Here's how the part is built. I have some questions about the finished solid (model axes, mm). A direction names the side the tool comes from. Give positions to 0.01 mm unless a question says otherwise; leave off trailing zeros. Order: outer loops, then holes, each group sorted by start corner. A loop starts at its lowest first (then second) coordinate and runs counter-clockwise, first axis right, second up.
from build123d import *
from build123d import SkipClean  # not in build123d's __all__

# Parameters (mm, degrees)
F2_R      = 1.25
F3_DEPTH  = 8.001
F5_R      = 1.25
F5_R_2    = 0.9
F6_DEPTH  = 3.2
F7_W      = 1
F7_H      = 4
F8_DEPTH  = 8
F9_R      = 0.9
F10_DEPTH = 2


with BuildPart() as f1:
    # F0 (on Right) → F1 (revolve)
    with BuildSketch(Plane.YZ):
        with BuildLine():
            Line((5, -0.8), (5, 0))
            ThreePointArc((5, 0), (3.5355339059, 3.5355339059), (0, 5))
            Line((0, 5), (0, -8))
            Line((0, -8), (1.7, -8))
            Line((1.7, -8), (1.7, 0))
            Line((1.7, 0), (4.6, 0))
            Line((4.6, 0), (4.6, -0.8))
            Line((4.6, -0.8), (5, -0.8))
        make_face()
    revolve(axis=Axis((0, 0, -1.5), (0, 0, -1)))

    # F2 (on Top) → F3 (cut, through all)
    with BuildSketch(Plane.XY):
        Circle(F2_R)
    extrude(amount=-F3_DEPTH, mode=Mode.SUBTRACT)

    # F5 (on face) → F6 (join)
    with BuildSketch(Plane(origin=(0, 0, 0), x_dir=(1, 0, 0), z_dir=(0, 0, -1))):
        Circle(F5_R)
        Circle(F5_R_2, mode=Mode.SUBTRACT)
    extrude(amount=F6_DEPTH)

    # F7 (on face) → F8 (cut, through all)
    with BuildSketch(Plane(origin=(0, 0, -8), x_dir=(1, 0, 0), z_dir=(0, 0, -1))):
        Rectangle(F7_W, F7_H)
    extrude(amount=-F8_DEPTH, mode=Mode.SUBTRACT)

    # F9 (on face) → F10 (cut)
    with BuildSketch(Plane(origin=(0, 0, 0), x_dir=(1, 0, 0), z_dir=(0, 0, -1))):
        Circle(F9_R)
    with SkipClean():  # cleaning this boolean's faces spoils the solid; the shape is the same uncleaned
        extrude(amount=-F10_DEPTH, mode=Mode.SUBTRACT)


solid = f1.part
Q1. I need wall thicknesses on L1, parallel to X at y = 0, z = -0.3; L2, parallel to X at y = 0, z = 0.65; L3, parallel to Y at x = 1.25, z = -0.25. Which ranges of each line are inside material? Lowest first, please.
Filled sheet:
L1: x = -5 to -4.6, -1.7 to -0.9, 0.9 to 1.7, 4.6 to 5
L2: x = -4.96 to -0.9, 0.9 to 4.96
L3: y = -4.84 to -4.43, -1.15 to 1.15, 4.43 to 4.84
Q2. If we section it at A-A on z = -1.5: List the corners of the cut face in (x, y) for me.
Filled sheet:
outline: (-0.5, -1.62) - (-0.5, -0.75) arc R0.9 cw to (-0.5, 0.75) - (-0.5, 1.62) arc R1.7 ccw to start; (0.5, -1.62) arc R1.7 ccw to (0.5, 1.62) - (0.5, 0.75) arc R0.9 cw to (0.5, -0.75) - close
Q3. If we section it at D-D on z = 1.25: List the corners of the cut face in (x, y) for me, plus the area to 3 significant figures.
Filled sheet:
outline: circle Ø9.68 at (0, 0); hole circle Ø1.8 at (0, 0)
area: 71.1 mm2
Q4. I'm going to push flat-ended pins straight in: P1, Ø0.8, axis at x = 1, y = -0.5, coming from the -Z side; P2, Ø0.7, axis at y = -1, z = -6, coming from the -X side; P3, Ø3, axis at x = -4, y = -3.5, coming from the +Z side; P4, Ø0.9, axis at x = -0.5, y = 0.5, coming from the -Z side. Where does each tip first touch, or does it pass through?
Filled sheet:
P1: stops at z = -8
P2: stops at x = -1.57
P3: stops at z = 3.23
P4: stops at z = -3.2
Q5. If we section it at B-B on x = 0: List the corners of the cut face in (y, z) for me.
Filled sheet:
outline: (-5, -0.8) - (-4.6, -0.8) - (-4.6, 0) - (-0.9, 0) - (-0.9, 2) - (0.9, 2) - (0.9, 0) - (4.6, 0) - (4.6, -0.8) - (5, -0.8) - (5, 0) arc R5 ccw to (-5, 0) - close
Q6. Thinking about a two-plate mould opening in Y: for faces 1 (the face through (1.25, -0.02, -5.57)), 2 (the face through (-4.88, -1.08, -0.39)), 3 (the face through (1.5, 0, -8)), which applies, released by +Y, released by -Y, zero draft, split by the parting line, or undercut?
Filled sheet:
face 1: undercut
face 2: split by the parting line
face 3: zero draft
Q7. If we section it at C-C on y = 0: List the corners of the cut face in (x, z) for me.
Filled sheet:
outline: (-5, -0.8) - (-4.6, -0.8) - (-4.6, 0) - (-1.7, 0) - (-1.7, -8) - (-1.25, -8) - (-1.25, -3.2) - (-0.9, -3.2) - (-0.9, 2) - (0.9, 2) - (0.9, -3.2) - (1.25, -3.2) - (1.25, -8) - (1.7, -8) - (1.7, 0) - (4.6, 0) - (4.6, -0.8) - (5, -0.8) - (5, 0) arc R5 ccw to (-5, 0) - close
Q8. For faces 4 (the face through (-2.8, -3.65, -0.41)), 5 (the face through (-1.5, 0, -8)), which set-ups out of +Z, -Z, +X, -X, +Y, -Y let a thin tool reach every point of the face, with its end or its side?
Filled sheet:
face 4: -Z
face 5: -Z, +X, -X, +Y, -Y
